Source: CAD feature listing. Evaluate the final solid. Frame: model axes, mm. Round coordinates to 2 decimals unless told otherwise and drop trailing zeros. Order: outer loops, then holes, each group sorted by start corner. A loop starts at its lowest first (then second) coordinate and runs counter-clockwise, first axis right, second up. Notation, with made-up numbers: (60.5, 73.25) - (72.5, 73.25) arc R24 ccw to (72.5, 88.25) - close; hole circle Ø11 at (43, 41). An arc over 180 degrees is marked (long way). Return JSON: item names as keys, results as strings. Group by question number.
1) Section A-A, the plane y = -2.4. Return loops of the section in (x, z), plus the area to 3 significant figures.
2) Section C-C, the plane z = -54.5. Return loops of the section in (x, y), plus the area to 3 significant figures.
3) Ray query, line 1 (X direction, y = -0.15, z = -84.5); line 2 (X direction, y = -2.1, z = -85); line 3 (Z direction, x = 34, y = -0.8). Return the intervals inside material, ascending. Write a range as from..to.
4) Contact query for flat-ended pins moving along their axis: P1, Ø1.5, axis at y = -2.5, z = 39, coming from the +X side; P2, Ø1.5, axis at y = -2.5, z = 39.5, coming from the +X side; P3, Ø3.5, axis at x = 48.75, z = -84.44, coming from the -Y side. Output: stop coordinate, or through.
5) Section B-B, the plane x = 27. Return loops of the section in (y, z).
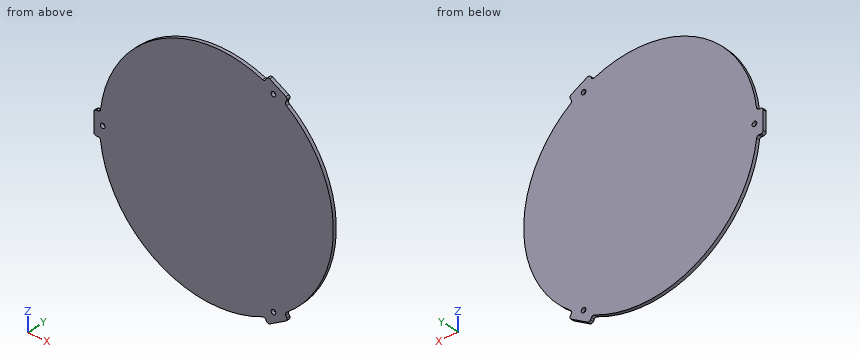
```python
from build123d import *

# Parameters (mm, degrees)
F0_R     = 2
F1_DEPTH = 3
F2_R     = 2
F3_R     = 2


with BuildPart() as f1:
    # F0 (on Front) → F1 (new body)
    with BuildSketch(Plane.XZ):
        with BuildLine():
            Line((-105, -10), (-99.498744, -10))
            ThreePointArc((-99.498744, -10), (-50, -86.60254), (41.089118, -91.16844))
            Line((41.089118, -91.16844), (43.839746, -95.932667))
            Line((43.839746, -95.932667), (61.160254, -85.932667))
            Line((61.160254, -85.932667), (58.409626, -81.16844))
            ThreePointArc((58.409626, -81.16844), (100, 0), (58.409626, 81.16844))
            Line((58.409626, 81.16844), (61.160254, 85.932667))
            Line((61.160254, 85.932667), (43.839746, 95.932667))
            Line((43.839746, 95.932667), (41.089118, 91.16844))
            ThreePointArc((41.089118, 91.16844), (-50, 86.60254), (-99.498744, 10))
            Line((-99.498744, 10), (-105, 10))
            Line((-105, 10), (-105, -10))
        make_face()
        with Locations((48.749372, -84.436389)):
            Circle(F0_R, mode=Mode.SUBTRACT)
        with Locations((-97.498744, 0)):
            Circle(F0_R, mode=Mode.SUBTRACT)
        with Locations((48.749372, 84.436389)):
            Circle(F0_R, mode=Mode.SUBTRACT)
    extrude(amount=F1_DEPTH)

    # F2
    f2_edges = [f1.edges().sort_by_distance(p)[0] for p in [
        (58.409626, -1.5, 81.16844),
        (41.089118, -1.5, 91.16844),
        (58.409626, -1.5, -81.16844),
        (41.089118, -1.5, -91.16844),
        (-99.498744, -1.5, -10),
        (-99.498744, -1.5, 10),
    ]]
    fillet(f2_edges, radius=F2_R)

    # F3
    f3_edges = [f1.edges().sort_by_distance(p)[0] for p in [
        (61.160254, -1.5, 85.932667),
        (43.839746, -1.5, 95.932667),
        (-105, -1.5, 10),
        (-105, -1.5, -10),
        (43.839746, -1.5, -95.932667),
        (61.160254, -1.5, -85.932667),
    ]]
    fillet(f3_edges, radius=F3_R)


solid = f1.part
```
Geometry check:
{
 "1": {"outline": "(-105, -8) arc R2 ccw to (-103, -10) - (-101.29, -10) arc R2 cw to (-99.31, -11.76) arc R100 ccw to (39.46, -91.88) arc R2 cw to (41.99, -92.72) - (42.84, -94.2) arc R2 ccw to (45.57, -94.93) - (59.43, -86.93) arc R2 ccw to (60.16, -84.2) - (59.31, -82.72) arc R2 cw to (59.84, -80.12) arc R100 ccw to (59.84, 80.12) arc R2 cw to (59.31, 82.72) - (60.16, 84.2) arc R2 ccw to (59.43, 86.93) - (45.57, 94.93) arc R2 ccw to (42.84, 94.2) - (41.99, 92.72) arc R2 cw to (39.46, 91.88) arc R100 ccw to (-99.31, 11.76) arc R2 cw to (-101.29, 10) - (-103, 10) arc R2 ccw to (-105, 8) - close; hole circle Ø4 at (-97.5, 0); hole circle Ø4 at (48.75, -84.44); hole circle Ø4 at (48.75, 84.44)", "area": "31,700 mm2"},
 "2": {"outline": "(-83.84, -3) - (83.84, -3) - (83.84, 0) - (-83.84, 0) - close", "area": "503 mm2"},
 "3": {"line 1": "-53.48..46.75, 50.75..60.3", "line 2": "-52.68..46.83, 50.67..60.42", "line 3": "-94.04..94.04"},
 "4": {"P1": "x = 92.4", "P2": "x = 92.19", "P3": "through"},
 "5": {"outline": "(-3, -96.29) - (0, -96.29) - (0, 96.29) - (-3, 96.29) - close"}
}
